Source: CAD feature listing. Evaluate the final solid. Frame: model axes, mm. A direction names the side the tool comes from. Round coordinates to 2 decimals unless told otherwise and drop trailing zeros. Loops run counter-clockwise (first coordinate to the right, second up) from the corner with the lowest first, then second, coordinate; pieces in that order, holes last.
(1) Mould query, pull axis X, two halves, no side actions, for faces 1 (the flat face through (-70, -406, 7)), 2 (the flat face through (-35, -30, 8)), 3 (the flat face through (-35, -800, 7)), 4 (the flat face through (0, -406, 7)). Classes: pulls with the +X half, pulls with the -X half, needs draft (parallel to the pull), parting line crosses it, or undercut.
(2) Section B-B, the plane y = -270. Return the cut outline in (x, z), plus the area to 3 significant figures.
(3) Section A-A, the plane z = 5.5. Return the cut outline in (x, y), plus the area to 3 significant figures.
(4) Material intervals for probe 1 along X at (y, z) = (-750, 2.25), sorted ascending.
(5) First-contact query: pin 1 Ø6 at (x, y) = (-35, -272.5) entering from -Z. Flat tip, straight axial feed; report the tip coordinate or a pass-through.
(6) Set-up query: faces 5 (the cylindrical face through (-32.83, -159.76, 3.94)), 6 (the flat face through (-35, 0, 7)). Return all of +Z, -Z, +X, -X, +Y, -Y with unobstructed straight access to the full face (end or side cutting, diameter ignored); none if empty.
```python
from build123d import *

# Parameters (mm, degrees)
SKETCH3_W           = 70
SKETCH3_H           = 800
BOSS_EXTRUDE1_DEPTH = 15
SKETCH4_R           = 10
CUT_EXTRUDE1_DEPTH  = 8


with BuildPart() as part:
    # Sketch3 → Boss-Extrude1 (new body)
    with BuildSketch(Plane.XY):
        with Locations((-35, -400)):
            Rectangle(SKETCH3_W, SKETCH3_H)
    extrude(amount=BOSS_EXTRUDE1_DEPTH)

    # Sketch4 → Cut-Extrude1 (cut)
    with BuildSketch(Plane(origin=(0, 0, 0), x_dir=(-1, 0, 0), z_dir=(0, 0, -1))):
        with Locations((35, -30)):
            Circle(SKETCH4_R)
        with Locations((35, -150)):
            Circle(SKETCH4_R)
        with Locations((35, -270)):
            Circle(SKETCH4_R)
        with Locations((35, -390)):
            Circle(SKETCH4_R)
        with Locations((35, -510)):
            Circle(SKETCH4_R)
        with Locations((35, -630)):
            Circle(SKETCH4_R)
        with Locations((35, -750)):
            Circle(SKETCH4_R)
    extrude(amount=-CUT_EXTRUDE1_DEPTH, mode=Mode.SUBTRACT)


solid = part.part
```
Output values:
1. face 1: pulls with the -X half
1. face 2: undercut
1. face 3: needs draft
1. face 4: pulls with the +X half
2. outline: (-70, 0) - (-45, 0) - (-45, 8) - (-25, 8) - (-25, 0) - (0, 0) - (0, 15) - (-70, 15) - close
2. area: 890 mm2
3. outline: (-70, -800) - (0, -800) - (0, 0) - (-70, 0) - close; hole circle Ø20 at (-35, -750); hole circle Ø20 at (-35, -630); hole circle Ø20 at (-35, -510); hole circle Ø20 at (-35, -390); hole circle Ø20 at (-35, -270); hole circle Ø20 at (-35, -150); hole circle Ø20 at (-35, -30)
3. area: 53,800 mm2
4. probe 1: x = -70 to -45, -25 to 0
5. pin 1: stops at z = 8
6. face 5: -Z
6. face 6: +Z, -Z, +X, -X, +Y
